Geometry check sheet. Reference: drawing and pictorial views, mm from the part's lowest x, y, z. A direction names the side the tool comes from. Round coordinates to 2 decimals unless told otherwise and drop trailing zeros. Order: outer loops, then holes, each group sorted by start corner. A loop starts at its lowest first (then second) coordinate and runs counter-clockwise, first axis right, second up. Notation, with made-up numbers: M 24.25,11 L 70.25,11 A29 cw 70.25,42 Z; hole C 41,1.25 d2. An arc over 180 degrees is marked long. Answer as a JSON object with one key per item and string values. Group by question number.
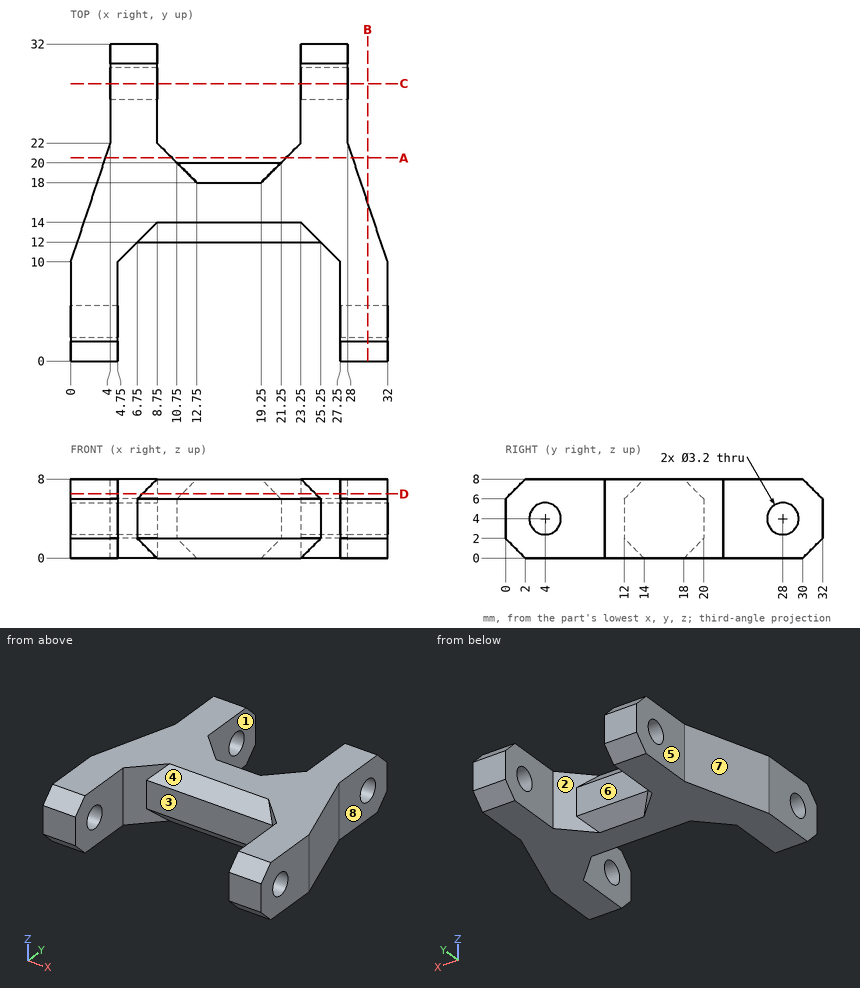
Q1. Thickness scan on line 1 (Z direction, x = 29.25, y = 4); line 2 (X direction, y = 26.5, z = 5.25); line 3 (X direction, y = 2, z = 2.25). Record the ranges inside material, lowest first. Write a range as from..to.
Q2. Tool access check on the marked faces 1, 2, 3, 4 and 5. Record the directions out of +Z, -Z, +X, -X, +Y, -Y that give a thin tool (end or side, any length) a straight path to the whole face; none if there is none.
Q3. Gauge pin test, flat ends, axial feed: pin 1 Ø2.5 at (y, z) = (4, 4) entering from +X; pin 2 Ø2.5 at (y, z) = (26.5, 3) entering from -X; pin 3 Ø3 at (x, z) = (18.5, 4.5) entering from +Y; pin 4 Ø3 at (x, z) = (15, 4) entering from -Y. Record the tip position at first contact, or that the pin passes through.
Q4. Release check for a two-part mould opening along X. For the marked faces 6, 7 and 8 record: released by +X, released by -X, zero draft, split by the parting line, or undercut.
Q5. Cross-section at D-D, the plane z = 6.5. Record the cut outline in (x, y), then the cut area to 4 significant figures.
Q6. Cross-section at C-C, the plane y = 28. Record the cut outline in (x, z), then the cut area to 3 significant figures.
Q7. Cross-section at A-A, the plane y = 20.5. Record the cut outline in (x, z), then the cut area to 3 significant figures.
Q8. Cross-section at B-B, the plane x = 30. Record the cut outline in (y, z).
Conclusion:
{
 "1": {"line 1": "0..2.4, 5.6..8", "line 2": "4..8.75, 23.25..28", "line 3": "0..4.75, 27.25..32"},
 "2": {"face 1": "+Z, -Z, +Y", "face 2": "+Y", "face 3": "+Z, -Z, -Y", "face 4": "+Z, -Y", "face 5": "+Z, -Z, -X, +Y"},
 "3": {"pin 1": "through", "pin 2": "x = 4", "pin 3": "y = 20", "pin 4": "y = 12"},
 "4": {"face 6": "undercut", "face 7": "released by -X", "face 8": "released by +X"},
 "5": {"outline": "M 0,0.5 L 4.75,0.5 L 4.75,10 L 7.25,12.5 L 24.75,12.5 L 27.25,10 L 27.25,0.5 L 32,0.5 L 32,10 L 28,22 L 28,31.5 L 23.25,31.5 L 23.25,22 L 20.75,19.5 L 11.25,19.5 L 8.75,22 L 8.75,31.5 L 4,31.5 L 4,22 L 0,10 Z", "area": "436.5 mm2"},
 "6": {"outline": "M 4,0 L 8.75,0 L 8.75,2.4 L 4,2.4 Z; M 4,5.6 L 8.75,5.6 L 8.75,8 L 4,8 Z; M 23.25,0 L 28,0 L 28,2.4 L 23.25,2.4 Z; M 23.25,5.6 L 28,5.6 L 28,8 L 23.25,8 Z", "area": "45.6 mm2"},
 "7": {"outline": "M 3.5,0 L 10.25,0 L 10.25,8 L 3.5,8 Z; M 21.75,0 L 28.5,0 L 28.5,8 L 21.75,8 Z", "area": "108 mm2"},
 "8": {"outline": "M 0,2 L 2,0 L 16,0 L 16,8 L 2,8 L 0,6 Z; hole C 4,4 d3.2"}
}
